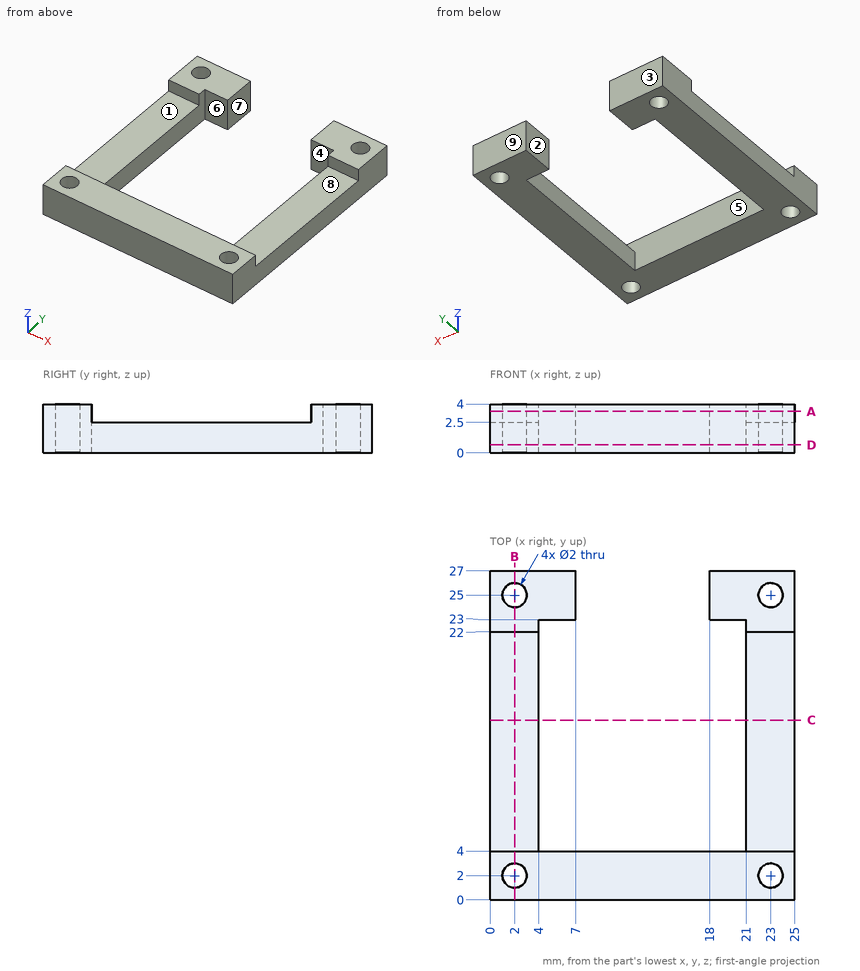
Check sheet for the drawn part. Datum: minimum x, y, z corner. Units: mm. A direction names the side the tool comes from. Coordinates: 2 decimals unless noted, no trailing zeros. Loops run counter-clockwise (first coordinate to the right, second up) from the corner with the lowest first, then second, coordinate; pieces in that order, holes last. Notation, with made-up numbers: (-33, -3.75) -> (23, -3.75) arc R23 cw to (23, 18.25) -> close; hole circle Ø7 at (88.5, 13). An arc over 180 degrees is marked (long way). Write each question's results on one line, items separated by ' | '.
Item 1: Section check B-B, the plane x = 2. Enter the section's corners in (y, z), plus the area to 3 significant figures.
Found:
outline: (0, 0) -> (1, 0) -> (1, 4) -> (0, 4) -> close; (3, 0) -> (24, 0) -> (24, 4) -> (22, 4) -> (22, 2.5) -> (4, 2.5) -> (4, 4) -> (3, 4) -> close; (26, 0) -> (27, 0) -> (27, 4) -> (26, 4) -> close | area: 65.0 mm2
Item 2: Section check C-C, the plane y = 14.75. Enter the section's corners in (x, z).
Found:
outline: (0, 0) -> (4, 0) -> (4, 2.5) -> (0, 2.5) -> close; (21, 0) -> (25, 0) -> (25, 2.5) -> (21, 2.5) -> close
Item 3: Section check A-A, the plane z = 3.4. Enter the section's corners in (x, y).
Found:
outline: (0, 0) -> (25, 0) -> (25, 4) -> (0, 4) -> close; (0, 22) -> (4, 22) -> (4, 23) -> (7, 23) -> (7, 27) -> (0, 27) -> close; (18, 23) -> (21, 23) -> (21, 22) -> (25, 22) -> (25, 27) -> (18, 27) -> close; hole circle Ø2 at (2, 2); hole circle Ø2 at (2, 25); hole circle Ø2 at (23, 2); hole circle Ø2 at (23, 25)
Item 4: Gauge pin test, flat ends, axial feed: pin 1 (1 mm diameter, centred on x = 22, y = 15, fed in from +Z); pin 2 (2 mm diameter, centred on x = 15, z = 2, fed in from -Y); pin 3 (2 mm diameter, centred on x = 13.5, z = 1.5, fed in from +Y). Record the tip position at first contact, or that the pin passes through.
Found:
pin 1: stops at z = 2.5 | pin 2: stops at y = 0 | pin 3: stops at y = 4
Item 5: Mould release check, pull along Y, two halves, no side actions. Record for the marked faces 1, 2, 3 and 4: +Y half, -Y half, draft (parallel to the pull), parting line (faces both ways), or undercut.
Found:
face 1: undercut | face 2: draft | face 3: +Y half | face 4: undercut
Item 6: Tool access check on the marked faces 5, 6, 7, 8 and 9. Record the directions out of +Z, -Z, +X, -X, +Y, -Y that give a thin tool (end or side, any length) a straight path to the whole face; none if there is none.
Found:
face 5: +Z | face 6: +Z, -Z | face 7: +Z, -Z, +Y | face 8: +Z, +X, -X | face 9: +Z, -Z, +X, -X, +Y
Item 7: Material ranges on L1, parallel to Y at x = 23, z = 2.25; L2, parallel to X at y = 25, z = 1.5; L3, parallel to X at y = 13.5, z = 2.05, recorded low to high.
Found:
L1: y = 0 to 1, 3 to 24, 26 to 27 | L2: x = 0 to 1, 3 to 7, 18 to 22, 24 to 25 | L3: x = 0 to 4, 21 to 25
Item 8: Section check D-D, the plane z = 0.65. Enter the section's corners in (x, y), plus the area to 3 significant figures.
Found:
outline: (0, 0) -> (25, 0) -> (25, 27) -> (18, 27) -> (18, 23) -> (21, 23) -> (21, 4) -> (4, 4) -> (4, 23) -> (7, 23) -> (7, 27) -> (0, 27) -> close; hole circle Ø2 at (2, 2); hole circle Ø2 at (2, 25); hole circle Ø2 at (23, 2); hole circle Ø2 at (23, 25) | area: 295 mm2
